```python
from build123d import *

# Parameters (mm, degrees)
F0_W     = 3.175
F0_H     = 76.2
F0_R     = 1.4605
F1_DEPTH = 6.35


with BuildPart() as f1:
    # F0 (on Front) → F1 (new body)
    with BuildSketch(Plane.XZ):
        Polygon((82.55, 12.7), (82.55, 44.45), (12.7, 44.45), (12.7, 38.1), (1.4605, 38.1), (1.4605, 33.655), (2.69367, 33.655), (2.69367, 31.115), (1.4605, 31.115), (1.4605, 26.67), (-1.4605, 26.67), (-1.4605, 31.115), (-2.69367, 31.115), (-2.69367, 33.655), (-1.4605, 33.655), (-1.4605, 38.1), (-12.7, 38.1), (-12.7, 44.45), (-82.55, 44.45), (-82.55, 12.7), (-88.9, 12.7), (-88.9, -12.7), (-82.55, -12.7), (-82.55, -44.45), (-12.7, -44.45), (-12.7, -38.1), (-1.4605, -38.1), (-1.4605, -33.655), (-2.69367, -33.655), (-2.69367, -31.115), (-1.4605, -31.115), (-1.4605, -26.67), (1.4605, -26.67), (1.4605, -31.115), (2.69367, -31.115), (2.69367, -33.655), (1.4605, -33.655), (1.4605, -38.1), (12.7, -38.1), (12.7, -44.45), (82.55, -44.45), (82.55, -12.7), (88.9, -12.7), (88.9, 12.7), align=None)
        with Locations((-75.301861, 0)):
            Rectangle(F0_W, F0_H, mode=Mode.SUBTRACT)
        with Locations((-68.951861, 0)):
            Rectangle(F0_W, F0_H, mode=Mode.SUBTRACT)
        with Locations((-62.601861, 0)):
            Rectangle(F0_W, F0_H, mode=Mode.SUBTRACT)
        with Locations((-56.251861, 0)):
            Rectangle(F0_W, F0_H, mode=Mode.SUBTRACT)
        with Locations((-49.901861, 0)):
            Rectangle(F0_W, F0_H, mode=Mode.SUBTRACT)
        with Locations((-43.551861, 0)):
            Rectangle(F0_W, F0_H, mode=Mode.SUBTRACT)
        with Locations((-37.201861, 0)):
            Rectangle(F0_W, F0_H, mode=Mode.SUBTRACT)
        with Locations((-30.851861, 0)):
            Rectangle(F0_W, F0_H, mode=Mode.SUBTRACT)
        with Locations((-85.725, 0)):
            Circle(F0_R, mode=Mode.SUBTRACT)
        with Locations((-23.0505, 0)):
            Circle(F0_R, mode=Mode.SUBTRACT)
        with Locations((23.0505, 0)):
            Circle(F0_R, mode=Mode.SUBTRACT)
        with Locations((30.486395, 0)):
            Rectangle(F0_W, F0_H, mode=Mode.SUBTRACT)
        with Locations((36.836395, 0)):
            Rectangle(F0_W, F0_H, mode=Mode.SUBTRACT)
        with Locations((43.186395, 0)):
            Rectangle(F0_W, F0_H, mode=Mode.SUBTRACT)
        with Locations((49.536395, 0)):
            Rectangle(F0_W, F0_H, mode=Mode.SUBTRACT)
        with Locations((55.886395, 0)):
            Rectangle(F0_W, F0_H, mode=Mode.SUBTRACT)
        with Locations((62.236395, 0)):
            Rectangle(F0_W, F0_H, mode=Mode.SUBTRACT)
        with Locations((68.586395, 0)):
            Rectangle(F0_W, F0_H, mode=Mode.SUBTRACT)
        with Locations((74.936395, 0)):
            Rectangle(F0_W, F0_H, mode=Mode.SUBTRACT)
        with Locations((85.725, 0)):
            Circle(F0_R, mode=Mode.SUBTRACT)
    extrude(amount=F1_DEPTH)


solid = f1.part
```
Can you work these out from the model? Positions are in its coordinate system, mm. A direction names the side the tool comes from. Coordinates: 2 decimals unless noted, no trailing zeros. Use a Markdown table: item, result.
Item 1: We'd pull the mould along X, two halves only. Please class faces 1 (the face through (-1.46, -3, 36)), 2 (the face through (48, -3, 44.45)): released by +X, released by -X, zero draft, split by the parting line, or undercut.
Numbers:
| item | result |
|---|---|
| face 1 | undercut |
| face 2 | zero draft |
Item 2: I want a section at A-A on z = 19. Give the number of separate pieces and of enclosed holes in the cut face, and give its area (3 significant figures).
Numbers:
| item | result |
|---|---|
| separate pieces | 17 |
| enclosed holes | 0 |
| area | 726 mm2 |
Item 3: Will these pins go through, and if not, where does the flat tip stop? pin 1 (4 mm diameter, centred on x = -23.05, z = 0, fed in from -Y); pin 2 (3 mm diameter, centred on y = -4.5, z = -41, fed in from +X); pin 3 (3 mm diameter, centred on y = -4.5, z = 26, fed in from -X).
Numbers:
| item | result |
|---|---|
| pin 1 | stops at y = -6.35 |
| pin 2 | stops at x = 82.55 |
| pin 3 | stops at x = -82.55 |
Item 4: If I drill on probe 1 along Z at (x, y) = (-57.5, -2.5); probe 2 along Z at (x, y) = (-10.5, -0.75), over which ranges is the centre line in solid material (lowest first)? Write a range as from..to.
Numbers:
| item | result |
|---|---|
| probe 1 | z = -44.45..-38.1, 38.1..44.45 |
| probe 2 | z = -38.1..38.1 |
Item 5: For faces 3 (the face through (47, -3, -44.45)), 4 (the face through (73.349, -3, -1)), 5 (the face through (86, -3, -12.7)), which set-ups out of +Z, -Z, +X, -X, +Y, -Y let a thin tool reach every point of the face, with its end or its side?
Numbers:
| item | result |
|---|---|
| face 3 | -Z, +X, -X, +Y, -Y |
| face 4 | +Y, -Y |
| face 5 | -Z, +X, +Y, -Y |
